```python
from build123d import *

# Parameters (mm, degrees)
SKIZZE1_W                       = 38.1
SKIZZE1_H                       = 38.1
SKIZZE1_W_2                     = 34.1
SKIZZE1_H_2                     = 34.1
AUFSATZ_LINEAR_AUSTRAGEN1_DEPTH = 3
SKIZZE2_W                       = 38.1
SKIZZE2_H                       = 38.1
AUFSATZ_LINEAR_AUSTRAGEN2_DEPTH = 15
VERRUNDUNG1_R                   = 5
VERRUNDUNG2_R                   = 7
SCHNITT_LINEAR_AUSTRAGEN1_DEPTH = 15


with BuildPart() as part:
    # Skizze1 → Aufsatz-Linear austragen1 (new body)
    with BuildSketch(Plane.XY):
        Rectangle(SKIZZE1_W, SKIZZE1_H)
        Rectangle(SKIZZE1_W_2, SKIZZE1_H_2, mode=Mode.SUBTRACT)
    extrude(amount=AUFSATZ_LINEAR_AUSTRAGEN1_DEPTH)

    # Skizze2 → Aufsatz-Linear austragen2 (add)
    with BuildSketch(Plane(origin=(0, 0, 0), x_dir=(-1, 0, 0), z_dir=(0, 0, -1))):
        Rectangle(SKIZZE2_W, SKIZZE2_H)
    extrude(amount=AUFSATZ_LINEAR_AUSTRAGEN2_DEPTH)

    # Verrundung1
    verrundung1_edges = [part.edges().sort_by_distance(p)[0] for p in [
        (-17.05, 17.05, 1.5),
        (-17.05, -17.05, 1.5),
        (17.05, -17.05, 1.5),
        (17.05, 17.05, 1.5),
    ]]
    fillet(verrundung1_edges, radius=VERRUNDUNG1_R)

    # Verrundung2
    verrundung2_edges = [part.edges().sort_by_distance(p)[0] for p in [
        (-19.05, 19.05, -6),
        (19.05, 19.05, -6),
        (19.05, -19.05, -6),
        (-19.05, -19.05, -6),
    ]]
    fillet(verrundung2_edges, radius=VERRUNDUNG2_R)

    # Skizze3 → Schnitt-Linear austragen1 (cut)
    with BuildSketch(Plane.XY):
        with BuildLine():
            Line((-13.05, 12.05), (-13.05, -12.05))
            ThreePointArc((-13.05, -12.05), (-12.757106781, -12.757106781), (-12.05, -13.05))
            Line((-12.05, -13.05), (12.05, -13.05))
            ThreePointArc((12.05, -13.05), (12.757106781, -12.757106781), (13.05, -12.05))
            Line((13.05, -12.05), (13.05, 12.05))
            ThreePointArc((13.05, 12.05), (12.757106781, 12.757106781), (12.05, 13.05))
            Line((12.05, 13.05), (-12.05, 13.05))
            ThreePointArc((-12.05, 13.05), (-12.757106781, 12.757106781), (-13.05, 12.05))
        make_face()
    extrude(amount=-SCHNITT_LINEAR_AUSTRAGEN1_DEPTH, mode=Mode.SUBTRACT)


solid = part.part
```
CAD build for the part. Positions are in the model's coordinates, mm. A direction names the side the tool comes from. Coordinates: 2 decimals unless noted, no trailing zeros. Loops run counter-clockwise (first coordinate to the right, second up) from the corner with the lowest first, then second, coordinate; pieces in that order, holes last. Notation, with made-up numbers: (13.25, -11) - (46.25, -11) arc R33 cw to (46.25, 25) - close; hole circle Ø9 at (49, 36.5). An arc over 180 degrees is marked (long way). Use CSV: the item, a comma, the result in double quotes. Start each with the question number.
Q1. 3-axis set-ups, long thin cutter, end or side, ignore diameter. For faces 5 (the flat face through (0, -17, -15)), 6 (the flat face through (-17.05, 0, 1)), 7 (the cylindrical face through (-12.765, -12.749, -7.395)): which of +Z, -Z, +X, -X, +Y, -Y reach the whole face in a straight line?
Q2. Cut at A-A, the plane y = 3. List the corners of the cut face in (x, z).
Q3. Cut at B-B, the plane z = -3.75. List the corners of the cut face in (x, y).
Q4. Probe probe 1 along X at (y, z) = (-7, -11.75); probe 2 along Z at (x, y) = (5, 17). List the from-to ranges inside material, lowest first. Write a range as from..to.
Q5. Cut at D-D, the plane x = -14. List the corners of the cut face in (y, z), then the cut area to 3 significant figures.
Q6. Two-plate mould, pull along X, no slides. Class faces 1 (the flat face through (0, 19.05, -6)), 2 (the flat face through (-19.05, 0, -6)), 3 (the cylindrical face through (17, -17, -6)), 4 (the flat face through (-15, 0, 0)): +X half, -X half, draft (parallel to the pull), parting line (faces both ways), or undercut.
Q7. Drop a flat-ended pin along its axis: P1, Ø5, axis at y = -15, z = -10.5, coming from the +X side. Give the stop position or say it passes through.
Here are the results:
1,face 5,"-Z, +X, -X, +Y, -Y"
1,face 6,"+Z"
1,face 7,"+Z, -Z"
2,outline,"(-19.05, -15) - (-13.05, -15) - (-13.05, 0) - (-17.05, 0) - (-17.05, 3) - (-19.05, 3) - close; (13.05, -15) - (19.05, -15) - (19.05, 3) - (17.05, 3) - (17.05, 0) - (13.05, 0) - close"
3,outline,"(-19.05, -12.05) arc R7 ccw to (-12.05, -19.05) - (12.05, -19.05) arc R7 ccw to (19.05, -12.05) - (19.05, 12.05) arc R7 ccw to (12.05, 19.05) - (-12.05, 19.05) arc R7 ccw to (-19.05, 12.05) - close; hole (-13.05, -12.05) arc R1 ccw to (-12.05, -13.05) - (12.05, -13.05) arc R1 ccw to (13.05, -12.05) - (13.05, 12.05) arc R1 ccw to (12.05, 13.05) - (-12.05, 13.05) arc R1 ccw to (-13.05, 12.05) - close"
4,probe 1,"-19.05..-13.05, 13.05..19.05"
4,probe 2,"-15..0"
5,outline,"(-18.77, -15) - (18.77, -15) - (18.77, 3) - (16.65, 3) - (16.65, 0) - (-16.65, 0) - (-16.65, 3) - (-18.77, 3) - close"
5,area,"576 mm2"
6,face 1,"draft"
6,face 2,"-X half"
6,face 3,"+X half"
6,face 4,"undercut"
7,P1,"x = 19.04"
